from build123d import *

# Parameters (mm, degrees)
SKETCH1_W           = 135
SKETCH1_H           = 83
SKETCH1_R           = 2.1
SKETCH1_R_2         = 8
SKETCH1_R_3         = 3
SKETCH1_R_4         = 4.725
SKETCH1_R_5         = 1.75
BOSS_EXTRUDE1_DEPTH = 5
SKETCH3_R           = 1
SKETCH3_W           = 23
SKETCH3_H           = 11.7
CUT_EXTRUDE1_DEPTH  = 80.394584198
FILLET1_R           = 8


with BuildPart() as part:
    # Sketch1 → Boss-Extrude1 (new body)
    with BuildSketch(Plane(origin=(0, 0, 0), x_dir=(1, 0, 0), z_dir=(0, 1, 0))):
        Rectangle(SKETCH1_W, SKETCH1_H)
        with Locations(Location((-9.98, 32.53, 0), (0, 0, 270))):
            Circle(SKETCH1_R, mode=Mode.SUBTRACT)
        with Locations(Location((55.08, 32.53, 0), (0, 0, 270))):
            Circle(SKETCH1_R, mode=Mode.SUBTRACT)
        with Locations(Location((55.08, -32.53, 0), (0, 0, 270))):
            Circle(SKETCH1_R, mode=Mode.SUBTRACT)
        with Locations(Location((-9.98, -32.53, 0), (0, 0, 270))):
            Circle(SKETCH1_R, mode=Mode.SUBTRACT)
        with Locations(Location((22.55, 0, 0), (0, 0, 270))):
            Circle(SKETCH1_R_2, mode=Mode.SUBTRACT)
        with Locations(Location((-46.455, 20.5, 0), (0, 0, 270))):
            Circle(SKETCH1_R_3, mode=Mode.SUBTRACT)
        with Locations(Location((-35.78, 0, 0), (0, 0, 270))):
            Circle(SKETCH1_R_4, mode=Mode.SUBTRACT)
        with Locations(Location((-46.455, -20.5, 0), (0, 0, 270))):
            Circle(SKETCH1_R_3, mode=Mode.SUBTRACT)
        with Locations(Location((-62.5, 36.5, 0), (0, 0, 270))):
            Circle(SKETCH1_R_5, mode=Mode.SUBTRACT)
        with Locations(Location((62.5, 36.5, 0), (0, 0, 270))):
            Circle(SKETCH1_R_5, mode=Mode.SUBTRACT)
        with Locations(Location((62.5, -36.5, 0), (0, 0, 270))):
            Circle(SKETCH1_R_5, mode=Mode.SUBTRACT)
        with Locations(Location((-62.5, -36.5, 0), (0, 0, 270))):
            Circle(SKETCH1_R_5, mode=Mode.SUBTRACT)
    extrude(amount=BOSS_EXTRUDE1_DEPTH)

    # Sketch3 → Cut-Extrude1 (cut, through all)
    with BuildSketch(Plane(origin=(0, 5, 0), x_dir=(1, 0, 0), z_dir=(0, 1, 0))):
        with Locations(Location((-27.43, 0, 0), (0, 0, 270))):
            Circle(SKETCH3_R)
        with Locations(Location((-56.43, 0, 0), (0, 0, 270))):
            Circle(SKETCH3_R)
        with Locations((-41.43, 0)):
            Rectangle(SKETCH3_W, SKETCH3_H)
    extrude(amount=-CUT_EXTRUDE1_DEPTH, mode=Mode.SUBTRACT)

    # Fillet1
    fillet1_edges = [part.edges().sort_by_distance(p)[0] for p in [
        (-67.5, 2.5, -41.5),
        (67.5, 2.5, -41.5),
        (67.5, 2.5, 41.5),
        (-67.5, 2.5, 41.5),
    ]]
    fillet(fillet1_edges, radius=FILLET1_R)


solid = part.part
Read the model definition and answer for the solid it produces. Units are mm, in the model's axes. A direction names the side the tool comes from. Round coordinates to 2 decimals unless told otherwise and drop trailing zeros. Order: outer loops, then holes, each group sorted by start corner. A loop starts at its lowest first (then second) coordinate and runs counter-clockwise, first axis right, second up. Notation, with made-up numbers: (72.5, 58) - (96.5, 58) arc R32 cw to (96.5, 91) - close; hole circle Ø10 at (-4.5, 42.5). An arc over 180 degrees is marked (long way). Use one line per item in the form item = value. Start each with the question number.
(1) For faces 4 (the face through (-65.219, 2.535, -39.094)), 5 (the face through (-42, 3, -5.85)), determine the directions among +Z, -Z, +X, -X, +Y, -Y from which every point of the face is accessible in a straight line to the end or side of a thin tool.
(2) The part is cut by section B-B (x = -35.5). Give the vertices of the cut face in (y, z).
(3) Find the intervals of material crossed by line 1 along X through (y, z) = (1.6, 0); line 2 along Z through (x, y) = (-56.5, 0.95); line 3 along X through (y, z) = (0.5, -20.5) (3 decimals), in increasing order. Write a range as from..to.
(4) The part is cut by section C-C (z = 36.5). Give the vertices of the cut face in (x, y), then the cut area to 3 significant figures.
(5) The part is cut by section A-A (z = 20.5). Give the vertices of the cut face in (x, y) (3 decimals), then the cut area to 3 significant figures.
(6) Determine the mould class of faces 1 (the face through (-64.21, 2.46, -36.88)), 2 (the face through (-1, 0, -1)), 3 (the face through (-65.219, 2.535, 39.094)) for opening direction X: +X half, -X half, draft (parallel to the pull), parting line (faces both ways), or undercut.
(7) The part is cut by section D-D (y = 3.1). Count the separate pieces of the cut face and the enclosed holes in it, then the cut area to 3 significant figures.
Checked values:
q1.face_4 = -Z, -X, +Y, -Y
q1.face_5 = +Y, -Y
q2.outline = (0, -41.5) - (5, -41.5) - (5, -5.85) - (0, -5.85) - close; (0, 5.85) - (5, 5.85) - (5, 41.5) - (0, 41.5) - close
q3.line_1 = -67.5..-57.43, -55.43..-52.93, -29.93..-28.43, -26.43..14.55, 30.55..67.5
q3.line_2 = -41.5..-1, 1..41.5
q3.line_3 = -67.5..-49.455, -43.455..67.5
q4.outline = (-66.92, 0) - (-64.25, 0) - (-64.25, 5) - (-66.92, 5) - close; (-60.75, 0) - (60.75, 0) - (60.75, 5) - (-60.75, 5) - close; (64.25, 0) - (66.92, 0) - (66.92, 5) - (64.25, 5) - close
q4.area = 634 mm^2
q5.outline = (-67.5, 0) - (-49.455, 0) - (-49.455, 5) - (-67.5, 5) - close; (-43.455, 0) - (67.5, 0) - (67.5, 5) - (-43.455, 5) - close
q5.area = 645 mm^2
q6.face_1 = undercut
q6.face_2 = draft
q6.face_3 = -X half
q7.separate_pieces = 1
q7.enclosed_holes = 14
q7.area = 10,500 mm^2
